Study the drawing (mm; zero at the part's minimum x, y, z) and answer. A direction names the side the tool comes from. Give positions to 0.01 mm unless a question says otherwise; leave off trailing zeros. Order: outer loops, then holes, each group sorted by start corner. A loop starts at its lowest first (then second) coordinate and runs counter-clockwise, first axis right, second up. Notation, with made-up numbers: (8.25, 57.25) - (64.25, 57.25) arc R23 cw to (64.25, 65.25) - close; hole circle Ø8 at (31.5, -2). An arc over 180 degrees is marked (long way). Use CSV: the item, a comma, the result in double quotes.
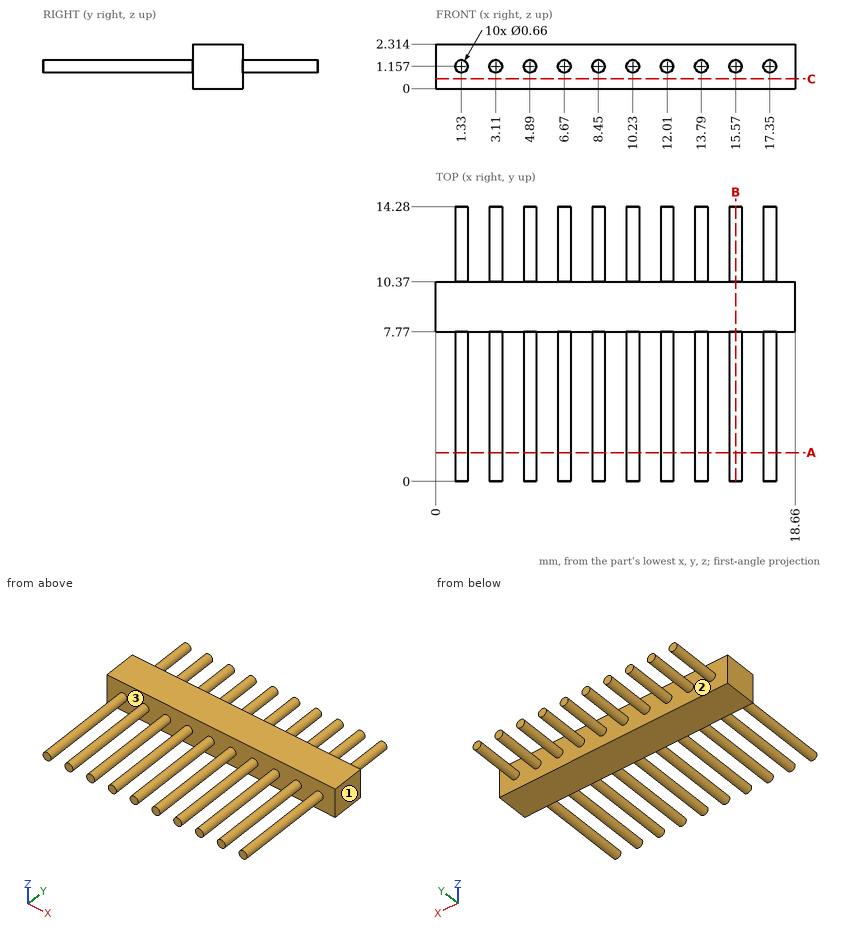
Item 1: The part is cut by section B-B (x = 15.57). Give the vertices of the cut face in (y, z).
Taken from the geometry:
outline,"(0, 0.83) - (7.77, 0.83) - (7.77, 0) - (10.37, 0) - (10.37, 0.83) - (14.28, 0.83) - (14.28, 1.49) - (10.37, 1.49) - (10.37, 2.31) - (7.77, 2.31) - (7.77, 1.49) - (0, 1.49) - close"
Item 2: The part is cut by section C-C (z = 0.5). Give the vertices of the cut face in (x, y), and give its area (3 significant figures).
Taken from the geometry:
outline,"(0, 7.77) - (18.66, 7.77) - (18.66, 10.37) - (0, 10.37) - close"
area,"48.5 mm^2"
Item 3: Which of the six approach directions +Z, -Z, +X, -X, +Y, -Y give full straight-line access (tool end or side, diameter ignored) to the marked faces 1, 2 and 3?
Taken from the geometry:
face 1,"+Z, -Z, +X, +Y, -Y"
face 2,"+Y"
face 3,"-Y"
Item 4: The part is cut by section A-A (y = 1.5). Count the separate pieces of the cut face and the enclosed holes in it, and give its area (3 significant figures).
Taken from the geometry:
separate pieces,"10"
enclosed holes,"0"
area,"3.42 mm^2"
Item 5: Find the intervals of material crossed by line 1 along Y through (x, z) = (10.75, 1.65); line 2 along Z through (x, y) = (12.25, 13.75); line 3 along Z through (x, y) = (17.25, 2.5), in increasing order.
Taken from the geometry:
line 1,"7.77 to 10.37"
line 2,"0.93 to 1.38"
line 3,"0.84 to 1.47"
